Design review of the part built by this model. Coordinates are the model's own, in mm. A direction names the side the tool comes from. Coordinates: 2 decimals unless noted, no trailing zeros. Loops run counter-clockwise (first coordinate to the right, second up) from the corner with the lowest first, then second, coordinate; pieces in that order, holes last. Notation, with made-up numbers: (70.25, 4.25) - (103.25, 4.25) arc R22 cw to (103.25, 30.25) - close; hole circle Ø1 at (73, -10). An arc over 180 degrees is marked (long way). Answer in a Markdown table with one row per item. Add a question column.
(1) We need section A-A, the plane x = 83. Write out the cut boundary in (y, z).
(2) To check wall thickness, follow L1, parallel to Z at x = 50, y = 22; L2, parallel to Y at x = 51.5, z = -33.5; L3, parallel to Z at x = 94, y = 21. State the ranges of each line that lie inside material, in increasing order. Write a range as [from, to].
(3) We need section D-D, the plane x = 26.5. Write out the cut boundary in (y, z), plus the area to 3 significant figures.
(4) For faces 1 (the face through (122, 5, -96)), 2 (the face through (121, 50, -187)), 3 (the face through (80, 25, -2)), list the 3-axis set-ups (+Z, -Z, +X, -X, +Y, -Y) from which the entire face can be reached by the end or side of a thin tool; tool diameter is ignored.
(5) We need section B-B, the plane y = 32. Write out the cut boundary in (x, z), plus the area to 3 significant figures.
(6) The part is to be moulded in two halves that separate along Z. For faces 4 (the face through (160, 25, -2)), 5 (the face through (217.95, 27.18, -96.26)), 6 (the face through (21.6, 27.2, -93.7)), 7 (the face through (119, 3, -5)), say which applies: released by +Z, released by -Z, zero draft, split by the parting line, or undercut.
(7) Clearance check with flat-ended pins moving along their axes: pin 1 (6 mm diameter, centred on y = 13.5, z = -40.5, fed in from +X); pin 2 (1.5 mm diameter, centred on y = 30.5, z = -3, fed in from -X); pin 3 (4 mm diameter, centred on y = 29.5, z = -135, fed in from +X). State where each tip first meets the part, or that it passes through.
(8) We need section C-C, the plane z = -100. Write out the cut boundary in (x, y).
from build123d import *

# Parameters (mm, degrees)
BOSS_EXTRUDE1_DEPTH = 50
SHELL2_T            = -5
SKETCH3_W           = 80
SKETCH3_H           = 50
CUT_EXTRUDE1_DEPTH  = 5


with BuildPart() as part:
    # Sketch1 → Boss-Extrude1 (new body)
    with BuildSketch(Plane(origin=(0, 0, 0), x_dir=(1, 0, 0), z_dir=(0, 1, 0))):
        Polygon((0, 0), (33.502126335, 190), (206.497873665, 190), (240, 0), align=None)
    extrude(amount=BOSS_EXTRUDE1_DEPTH)

    # Shell2
    shell2_openings = [part.faces().sort_by_distance(p)[0] for p in [
        (120, 50, -95),
    ]]
    offset(amount=SHELL2_T, openings=shell2_openings, kind=Kind.INTERSECTION)

    # Sketch3 → Cut-Extrude1 (cut)
    with BuildSketch(Plane.XY):
        with Locations((120, 25)):
            Rectangle(SKETCH3_W, SKETCH3_H)
    extrude(amount=-CUT_EXTRUDE1_DEPTH, mode=Mode.SUBTRACT)


solid = part.part
Responses:
| question | item | result |
|---|---|---|
| 1 | outline | (0, -190) - (50, -190) - (50, -185) - (5, -185) - (5, -5) - (0, -5) - close |
| 2 | L1 | z = [-190, -185], [-5, 0] |
| 2 | L2 | y = [0, 5] |
| 2 | L3 | z = [-190, -185] |
| 3 | outline | (0, -150.29) - (50, -150.29) - (50, -121.5) - (5, -121.5) - (5, -5) - (50, -5) - (50, 0) - (0, 0) - close |
| 3 | area | 2,270 mm2 |
| 4 | face 1 | +Y |
| 4 | face 2 | +Z, -Z, +X, -X, +Y |
| 4 | face 3 | +Z, +Y, -Y |
| 5 | outline | (0, 0) - (33.5, -190) - (206.5, -190) - (240, 0) - (160, 0) - (160, -5) - (234.04, -5) - (202.3, -185) - (37.7, -185) - (5.96, -5) - (80, -5) - (80, 0) - close |
| 5 | area | 3,490 mm2 |
| 6 | face 4 | zero draft |
| 6 | face 5 | undercut |
| 6 | face 6 | undercut |
| 6 | face 7 | released by +Z |
| 7 | pin 1 | stops at x = 233.39 |
| 7 | pin 2 | stops at x = 0.4 |
| 7 | pin 3 | stops at x = 216.55 |
| 8 | outline | (17.63, 0) - (222.37, 0) - (222.37, 50) - (217.29, 50) - (217.29, 5) - (22.71, 5) - (22.71, 50) - (17.63, 50) - close |
